from build123d import *

# Parameters (mm, degrees)
BOSS_EXTRUDE1_DEPTH = 3.5
FILLET1_R           = 4
SKETCH2_R           = 1.75
CUT_EXTRUDE1_DEPTH  = 63.747509911
CUT_EXTRUDE2_DEPTH  = 63.747509911
LPATTERN1_COUNT     = 5
LPATTERN1_PITCH     = 10
LPATTERN1_COL_COUNT = 5
LPATTERN1_COL_PITCH = 10


with BuildPart() as part:
    # Sketch1 → Boss-Extrude1 (new body)
    with BuildSketch(Plane.XY):
        Polygon((-55, 20), (-40, 20), (-30, 30), (30, 30), (40, 20), (55, 20), (55, -20), (40, -20), (30, -30), (-30, -30), (-40, -20), (-55, -20), align=None)
    extrude(amount=BOSS_EXTRUDE1_DEPTH)

    # Fillet1
    fillet1_edges = [part.edges().sort_by_distance(p)[0] for p in [
        (-55, -20, 1.75),
        (-55, 20, 1.75),
        (-40, 20, 1.75),
        (-30, 30, 1.75),
        (30, 30, 1.75),
        (40, 20, 1.75),
        (55, 20, 1.75),
        (55, -20, 1.75),
        (40, -20, 1.75),
        (30, -30, 1.75),
        (-30, -30, 1.75),
        (-40, -20, 1.75),
    ]]
    fillet(fillet1_edges, radius=FILLET1_R)

    # Sketch2 → Cut-Extrude1 (cut, through all)
    with BuildSketch(Plane.XY.offset(3.5)):
        with Locations((-50, 15)):
            Circle(SKETCH2_R)
        with Locations((-50, -15)):
            Circle(SKETCH2_R)
        with Locations((50, -15)):
            Circle(SKETCH2_R)
        with Locations((50, 15)):
            Circle(SKETCH2_R)
    extrude(amount=-CUT_EXTRUDE1_DEPTH, mode=Mode.SUBTRACT)

    # Sketch3 → Cut-Extrude2 (cut, through all)
    with BuildSketch(Plane.XY.offset(3.5)):
        with BuildLine():
            Line((-0.25, 14), (0.25, 14))
            ThreePointArc((0.25, 14), (0.957106781, 13.707106781), (1.25, 13))
            Line((1.25, 13), (1.25, -13))
            ThreePointArc((1.25, -13), (0.957106781, -13.707106781), (0.25, -14))
            Line((0.25, -14), (-0.25, -14))
            ThreePointArc((-0.25, -14), (-0.957106781, -13.707106781), (-1.25, -13))
            Line((-1.25, -13), (-1.25, 13))
            ThreePointArc((-1.25, 13), (-0.957106781, 13.707106781), (-0.25, 14))
        make_face()
    cut_extrude2 = extrude(amount=-CUT_EXTRUDE2_DEPTH, mode=Mode.SUBTRACT)

    # LPattern1: Cut-Extrude2 ×5
    with Locations(*[(-i * LPATTERN1_PITCH, 0, 0) for i in range(1, LPATTERN1_COUNT)]):
        add(cut_extrude2, mode=Mode.SUBTRACT)

    # LPattern1 col: Cut-Extrude2 ×5
    with Locations(*[(i * LPATTERN1_COL_PITCH, 0, 0) for i in range(1, LPATTERN1_COL_COUNT)]):
        add(cut_extrude2, mode=Mode.SUBTRACT)


solid = part.part
Geometry: final body of the model. Coordinates: model frame, mm. A direction names the side the tool comes from. Coordinates: 2 decimals unless noted, no trailing zeros. Loops run counter-clockwise (first coordinate to the right, second up) from the corner with the lowest first, then second, coordinate; pieces in that order, holes last. Notation, with made-up numbers: (77.25, 52) - (104.25, 52) arc R22 ccw to (104.25, 67) - close; hole circle Ø5 at (54.25, -29.75). An arc over 180 degrees is marked (long way). Put each result on its own line as item: value. Start each with the question number.
Q1. Pin query (flat end, axial travel): pin 1 Ø4.5 at (x, y) = (-50, -15) entering from +Z; pin 2 Ø1.8 at (x, z) = (-45.5, 1.5) entering from -Y. Return the tip coordinate at first contact, or that it passes through.
Q2. Pull-direction query (Y, two-part tool) for faces 1 (the cylindrical face through (-48.331, -14.474, 1.774)), 2 (the flat face through (-11.5, 0.4, 3.5)), 3 (the flat face through (18.75, 0, 2)), 4 (the flat face through (0, -30, 2)); classes: released by +Y, released by -Y, zero draft, split by the parting line, or undercut.
Q3. Cut plane C-C, the plane x = -44. Return loops of the section in (y, z), and give its area (3 significant figures).
Q4. Cut plane A-A, the plane z = 2.1. Give the number of separate pieces and of enclosed holes in the cut face, and give its area (3 significant figures).
Q5. Set-up query: faces 5 (the flat face through (28.75, 0, 2)), 6 (the flat face through (46, 20, 2)), 7 (the cylindrical face through (53.859, -18.797, 1.774)). Return all of +Z, -Z, +X, -X, +Y, -Y with unobstructed straight access to the full face (end or side cutting, diameter ignored); none if empty.
Q6. Line query: line 1 (Y direction, x = -50, z = 1.15); line 2 (X direction, y = 16, z = 2.1); line 3 (Y direction, x = 49, z = 0.2). Output: solid intervals per line, ascending.
Q7. Cut plane B-B, the plane y = -22.5. Return loops of the section in (x, z).
Filled sheet:
1. pin 1: z = 3.5
1. pin 2: y = -20
2. face 1: undercut
2. face 2: zero draft
2. face 3: undercut
2. face 4: released by -Y
3. outline: (-20, 0) - (20, 0) - (20, 3.5) - (-20, 3.5) - close
3. area: 140 mm²
4. separate pieces: 1
4. enclosed holes: 13
4. area: 5,130 mm²
5. face 5: +Z, -Z
5. face 6: +Z, -Z, +X, +Y
5. face 7: +Z, -Z, +X, -Y
6. line 1: -20 to -16.75, -13.25 to 13.25, 16.75 to 20
6. line 2: -55 to -51.44, -48.56 to 48.56, 51.44 to 55
6. line 3: -20 to -16.44, -13.56 to 13.56, 16.44 to 20
7. outline: (-37.5, 0) - (37.5, 0) - (37.5, 3.5) - (-37.5, 3.5) - close
